Work out the finished part from the listing and answer in its coordinate system (mm). Give positions to 0.01 mm unless a question says otherwise; leave off trailing zeros. Write each loop counter-clockwise with the first axis right and the second up, starting at its lowest first coordinate (ties: lowest second). Pieces come first, ordered by that corner, then holes. Notation, with made-up numbers: (-21.75, 23.5) -> (-7.75, 23.5) arc R32 cw to (-7.75, 58.5) -> close; hole circle Ø6 at (79.25, -21). An arc over 180 degrees is marked (long way). Use a Markdown table: item, result. Add a question column.
Q1. Consider line 1 (X direction, y = 67, z = -5.5); line 2 (Y direction, x = -52, z = -3); line 3 (X direction, y = 26, z = -2.25). Determine where each line is inside the solid, lowest interval first.
Q2. Section A-A, the plane z = -4.5 is taken. Give the vertices of the cut face in (x, y).
Q3. Each of these flat-tipped pins is pushed along its axis until it touches: pin 1 Ø3 at (y, z) = (13, -3.5) entering from +X; pin 2 Ø1.5 at (y, z) = (32, -5) entering from -X; pin 3 Ø3 at (y, z) = (48.5, -3) entering from +X. Where does it stop, or does it pass through?
Q4. Section B-B, the plane x = -45 is taken. Give the vertices of the cut face in (y, z).
Q5. Section C-C, the plane y = -54 is taken. Give the vertices of the cut face in (x, z), plus the area to 3 significant figures.
from build123d import *

# Parameters (mm, degrees)
F1_DEPTH = 6.35


with BuildPart() as f1:
    # F0 (on Top) → F1 (new body)
    with BuildSketch(Plane.XY):
        with BuildLine():
            ThreePointArc((-105, -36.5), (-103.140128, -40.990128), (-98.65, -42.85))
            Line((-98.65, -42.85), (-19.05, -42.85))
            ThreePointArc((-19.05, -42.85), (-5.579616, -48.429616), (0, -61.9))
            Line((0, -61.9), (0, -80.95))
            ThreePointArc((0, -80.95), (5.579616, -94.420384), (19.05, -100))
            Line((19.05, -100), (92.65, -100))
            ThreePointArc((92.65, -100), (97.140128, -98.140128), (99, -93.65))
            Line((99, -93.65), (99, -63.117434))
            ThreePointArc((99, -63.117434), (98.377326, -60.375129), (96.631422, -58.170639))
            ThreePointArc((96.631422, -58.170639), (68.778704, 0), (96.631422, 58.170639))
            ThreePointArc((96.631422, 58.170639), (98.377326, 60.375129), (99, 63.117434))
            Line((99, 63.117434), (99, 93.65))
            ThreePointArc((99, 93.65), (97.140128, 98.140128), (92.65, 100))
            Line((92.65, 100), (21.65, 100))
            ThreePointArc((21.65, 100), (8.179616, 94.420384), (2.6, 80.95))
            Line((2.6, 80.95), (2.6, 75.15))
            Line((2.6, 75.15), (2.6, 31.5))
            ThreePointArc((2.6, 31.5), (0.740128, 27.009872), (-3.75, 25.15))
            Line((-3.75, 25.15), (-29.15, 25.15))
            ThreePointArc((-29.15, 25.15), (-33.640128, 27.009872), (-35.5, 31.5))
            Line((-35.5, 31.5), (-35.5, 68.8))
            ThreePointArc((-35.5, 68.8), (-37.359872, 73.290128), (-41.85, 75.15))
            Line((-41.85, 75.15), (-98.65, 75.15))
            ThreePointArc((-98.65, 75.15), (-103.140128, 73.290128), (-105, 68.8))
            Line((-105, 68.8), (-105, 50.309879))
            ThreePointArc((-105, 50.309879), (-103.727052, 46.495952), (-100.41857, 44.211136))
            ThreePointArc((-100.41857, 44.211136), (-79.338794, 16.15), (-100.41857, -11.911136))
            ThreePointArc((-100.41857, -11.911136), (-103.727052, -14.195952), (-105, -18.009879))
            Line((-105, -18.009879), (-105, -36.5))
        make_face()
    extrude(amount=-F1_DEPTH)


solid = f1.part
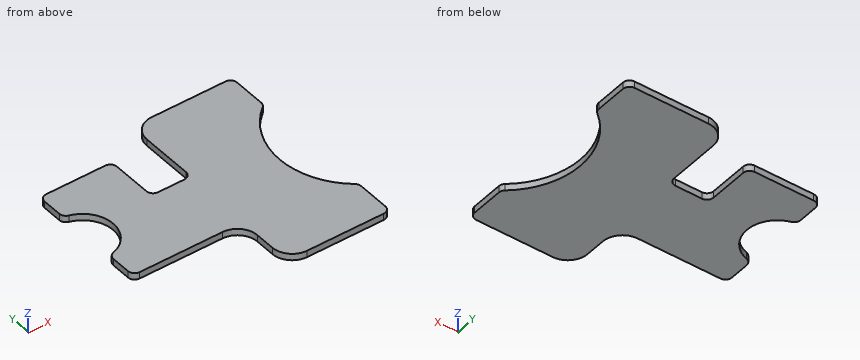
Result set:
| question | item | result |
|---|---|---|
| 1 | line 1 | x = -105 to -35.5, 2.6 to 99 |
| 1 | line 2 | y = -42.85 to 75.15 |
| 1 | line 3 | x = -81.05 to -32.32, -0.58 to 73.45 |
| 2 | outline | (-105, -36.5) arc R6.35 ccw to (-98.65, -42.85) -> (-19.05, -42.85) arc R19.05 cw to (0, -61.9) -> (0, -80.95) arc R19.05 ccw to (19.05, -100) -> (92.65, -100) arc R6.35 ccw to (99, -93.65) -> (99, -63.12) arc R6.35 ccw to (96.63, -58.17) arc R74.67 cw to (96.63, 58.17) arc R6.35 ccw to (99, 63.12) -> (99, 93.65) arc R6.35 ccw to (92.65, 100) -> (21.65, 100) arc R19.05 ccw to (2.6, 80.95) -> (2.6, 31.5) arc R6.35 cw to (-3.75, 25.15) -> (-29.15, 25.15) arc R6.35 cw to (-35.5, 31.5) -> (-35.5, 68.8) arc R6.35 ccw to (-41.85, 75.15) -> (-98.65, 75.15) arc R6.35 ccw to (-105, 68.8) -> (-105, 50.31) arc R6.35 ccw to (-100.42, 44.21) arc R29.22 cw to (-100.42, -11.91) arc R6.35 ccw to (-105, -18.01) -> close |
| 3 | pin 1 | stops at x = 70.2 |
| 3 | pin 2 | stops at x = -84.51 |
| 3 | pin 3 | stops at x = 87.99 |
| 4 | outline | (-42.85, -6.35) -> (75.15, -6.35) -> (75.15, 0) -> (-42.85, 0) -> close |
| 5 | outline | (-1.72, -6.35) -> (91.88, -6.35) -> (91.88, 0) -> (-1.72, 0) -> close |
| 5 | area | 594 mm2 |
